Build history of the part. All positions in model axes, mm. Face numbers are marked on the shaded views. A direction names the side the tool comes from. Round coordinates to 2 decimals unless told otherwise and drop trailing zeros. Write each loop counter-clockwise with the first axis right and the second up, starting at its lowest first coordinate (ties: lowest second). Pieces come first, ordered by that corner, then holes. Notation, with made-up numbers: (52, 28.25) - (98, 28.25) arc R24 cw to (98, 59.25) - close; hole circle Ø11 at (-16, -15.75). An arc over 180 degrees is marked (long way). Answer as a JSON object with one key per item and string values. Group by question number.
Item 1: Slice it at C-C, the plane z = 3. List the corners of the cut face in (x, y).
Item 2: Two-plate mould, pull along Z, no slides. Class the marked faces 3, 4 and 5: +Z half, -Z half, draft (parallel to the pull), parting line (faces both ways), or undercut.
Item 3: Slice it at A-A, the plane y = 3. List the corners of the cut face in (x, z), then the cut area to 3 significant figures.
Item 4: Slice it at B-B, the plane x = -0.9. Give the number of separate pieces and of enclosed holes in the cut face, then the cut area to 3 significant figures.
Item 5: Probe line 1 (Z direction, x = 0.3, y = 3); line 2 (Y direction, x = -1.05, z = 0); line 3 (Z direction, x = 0.35, y = 22.5). List the from-to ranges inside material, lowest first. Write a range as from..to.
Item 6: Which spindle directions (+Z, -Z, +X, -X, +Y, -Y) get a long thin tool onto all of the face, cutting with end or side? Do the marked faces 1 and 2. Say none if no direction does.
Item 7: Flat gauge pins, fed straight in: pin 1 (1.2 mm diameter, centred on y = 3, z = -3, fed in from -X); pin 2 (1 mm diameter, centred on y = 19, z = 2.5, fed in from +X). Where does each tip first touch, or does it go through?
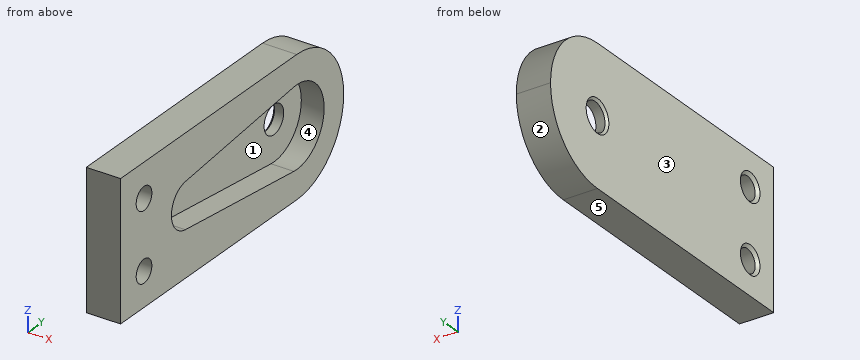
Autodesk Inventor part; units mm, degrees
ref_plane "YZ Plane" through (0, 0, 0) normal (1, 0, 0) x (0, 1, 0)
ref_plane "XZ Plane" through (0, 0, 0) normal (0, 1, 0) x (-1, 0, 0)
ref_plane "XY Plane" through (0, 0, 0) normal (0, 0, 1) x (1, 0, 0)
sketch "Sketch1" plane through (0, 0, 0) normal (0, 1, 0) x (-1, 0, 0)
  line L0 (-1.5, 6) -> (1.5, 6)
  line L1 (1.5, 6) -> (1.5, -6)
  line L2 (1.5, -6) -> (-1.5, -6)
  line L3 (-1.5, -6) -> (-1.5, 6)
  line L4 (-1.5, 6) -> (1.5, -6) construction
  line L5 (1.5, 6) -> (-1.5, -6) construction
  point P0 (0, 0)
  dimension "d0" = 3
  dimension "d1" = 12
extrude "Extrusion1" add sketch "Sketch1" along normal blind 28.5
fillet "Fillet1" radius 6 2 edges at (0, 28.5, 6) (0, 28.5, -6)
sketch "Sketch3" plane through (1.5, 0, 6) normal (1, 0, 0) x (0, 0, -1)
  arc A0 (12, 22.5) -> (0, 22.5) centre (6, 22.5) ccw
  arc A1 (9.4799, 22.125) -> (2.5201, 22.125) centre (6, 22.5) ccw
  line L0 (6, 22.5) -> (6, 8.5) construction
  line L1 (6, 22.5) -> (20, 22.5) construction
  arc A2 (4.0115, 8.2857) -> (7.9885, 8.2857) centre (6, 8.5) ccw
  line L2 (4.0115, 8.2857) -> (2.5201, 22.125)
  line L3 (7.9885, 8.2857) -> (9.4799, 22.125)
  circle A3 centre (6, 22.5) radius 1.25
  point P0 (6, 0)
  dimension "d8" = 7
  dimension "d9" = 14
  dimension "d10" = 90
  dimension "d11" = 4
  dimension "d43" = 2.5
extrude "Extrusion3" cut sketch "Sketch3" against normal blind 2
sketch "Sketch6" plane through (-1.5, 0, -6) normal (-1, 0, 0) x (0, 0, 1)
  line L0 (6, 0) -> (6, 28.5)
  arc A0 (12, 22.5) -> (0, 22.5) centre (6, 22.5) ccw
  line L1 (0, 0) -> (12, 0) construction
  line L2 (0, 0) -> (3, 0) construction
  line L3 (3, 0) -> (3, 3) construction
  line L4 (3, 3) -> (0, 3) construction
  line L5 (0, 3) -> (0, 0) construction
  line L6 (9, 0) -> (9, 3) construction
  line L7 (9, 3) -> (12, 3) construction
  dimension "d35" = 3
hole "Hole2" at (-1.5, 3, -3) at (-1.5, 3, 3) direction (1, 0, 0) diameter 2 depth 3 countersink diameter 2.5 countersink angle 90
extrude "Vysunutí6" cut sketch "Sketch3" against normal through all contours A3
chamfer "Chamfer1" distance 0.2 angle 45 1 edges at (-1.5, 22.5, 1.25)
properties part number "middleLegv2-2_3DPrint"
Geometry says:
{
 "1": {"outline": "(-1.5, 0) - (1.5, 0) - (1.5, 2) - (-1.25, 2) - (-1.5, 1.75) - close; (-1.5, 4.25) - (-1.25, 4) - (1.5, 4) - (1.5, 17.67) - (-0.5, 17.67) - (-0.5, 24.3) - (1.5, 24.3) - (1.5, 27.7) - (-1.5, 27.7) - close"},
 "2": {"face 3": "draft", "face 4": "undercut", "face 5": "-Z half"},
 "3": {"outline": "(-1.5, -6) - (1.5, -6) - (1.5, -4) - (-1.25, -4) - (-1.5, -4.25) - close; (-1.5, -1.75) - (-1.25, -2) - (1.5, -2) - (1.5, 2) - (-1.25, 2) - (-1.5, 1.75) - close; (-1.5, 4.25) - (-1.25, 4) - (1.5, 4) - (1.5, 6) - (-1.5, 6) - close", "area": "23.9 mm^2"},
 "4": {"separate pieces": "1", "enclosed holes": "3", "area": "315 mm^2"},
 "5": {"line 1": "z = -6..-4, -2..2, 4..6", "line 2": "y = 0..21.25, 23.75..28.5", "line 3": "z = -6..-3.5, 3.5..6"},
 "6": {"face 1": "+X", "face 2": "-Z, +X, -X, +Y"},
 "7": {"pin 1": "passes through", "pin 2": "stops at x = -0.5"}
}
